Verification items for the finished model (mm, model axes). A direction names the side the tool comes from. Coordinates: 2 decimals unless noted, no trailing zeros. Write each loop counter-clockwise with the first axis right and the second up, starting at its lowest first coordinate (ties: lowest second). Pieces come first, ordered by that corner, then holes. Notation, with made-up numbers: (84, 88) -> (138, 88) arc R27 ccw to (138, 127) -> close; hole circle Ø3 at (18, 54.5). An arc over 180 degrees is marked (long way). Write item = value, one per line. Start each with the question number.
(1) Mould release check, pull along X, two halves, no side actions. Record for faces 4 (the face through (7, 35, 15)), 5 (the face through (0, 35, 15)), 6 (the face through (101, 36, 33.15)): released by +X, released by -X, zero draft, split by the parting line, or undercut.
(2) Material ranges on probe 1 along X at (y, z) = (58, 13); probe 2 along Z at (x, y) = (34.5, 14); probe 3 along Z at (x, y) = (4.5, 44), recorded low to high. Write a range as [from, to].
(3) Section check A-A (y = 28.5). Record the cut outline in (x, z).
(4) Section check B-B (z = 25). Record the cut outline in (x, y).
(5) Gauge pin test, flat end, axial feed: pin 1 Ø9 at (y, z) = (25.5, 13) entering from +X. Record the tip position at first contact, or that the pin passes through.
(6) Section check C-C (x = 142.5). Record the cut outline in (y, z).
(7) Section check D-D (z = 13). Record the cut outline in (x, y), plus the area to 3 significant figures.
(8) Set-up check for faces 1 (the face through (198, 35, 15)), 2 (the face through (205, 35, 15)), 3 (the face through (102, 0, 31)): record each of +Z, -Z, +X, -X, +Y, -Y from which the full face is reachable in a straight line by a thin tool's end or side.
```python
from build123d import *

# Parameters (mm, degrees)
SKETCH_1_W        = 7
SKETCH_1_H        = 70
EXTRUDE_1_DEPTH   = 30.15
EXTRUDE_1_2_DEPTH = 30.15
FILLET_1_R        = 30
FILLET_2_R        = 30
SKETCH_2_W        = 215.9
SKETCH_2_H        = 71
EXTRUDE_2_DEPTH   = 3
FILLET_3_R        = 3


with BuildPart() as part:
    # Sketch 1 → Extrude 1 (new body)
    with BuildSketch(Plane.XY):
        with Locations((3.5, 35)):
            Rectangle(SKETCH_1_W, SKETCH_1_H)
    extrude(amount=EXTRUDE_1_DEPTH)

    # Fillet 2
    fillet_2_edges = [part.edges().sort_by_distance(p)[0] for p in [
        (3.5, 70, 0),
    ]]
    fillet(fillet_2_edges, radius=FILLET_2_R)



with BuildPart() as body_2:
    # Sketch 1 → Extrude 1 2 (new body)
    with BuildSketch(Plane.XY):
        with Locations((201.5, 35)):
            Rectangle(SKETCH_1_W, SKETCH_1_H)
    extrude(amount=EXTRUDE_1_2_DEPTH)

    # Fillet 1
    fillet_1_edges = [body_2.edges().sort_by_distance(p)[0] for p in [
        (201.5, 70, 0),
    ]]
    fillet(fillet_1_edges, radius=FILLET_1_R)


with BuildPart() as part_1:
    add(part.part)

    add(body_2.part)  # Extrude 2 merges body 2
    # Sketch 2 → Extrude 2 (add)
    with BuildSketch(Plane.XY.offset(30.15)):
        with Locations((102.5, 35.5)):
            Rectangle(SKETCH_2_W, SKETCH_2_H)
    extrude(amount=EXTRUDE_2_DEPTH)

    # Fillet 3
    fillet_3_edges = [part_1.edges().sort_by_distance(p)[0] for p in [
        (210.45, 0, 31.65),
        (210.45, 71, 31.65),
        (-5.45, 71, 31.65),
        (-5.45, 0, 31.65),
    ]]
    fillet(fillet_3_edges, radius=FILLET_3_R)


solid = part_1.part
```
Response:
q1.face_4 = undercut
q1.face_5 = released by -X
q1.face_6 = zero draft
q2.probe_1 = [0, 7], [198, 205]
q2.probe_2 = [30.15, 33.15]
q2.probe_3 = [0.27, 33.15]
q3.outline = (-5.45, 30.15) -> (0, 30.15) -> (0, 0) -> (7, 0) -> (7, 30.15) -> (198, 30.15) -> (198, 0) -> (205, 0) -> (205, 30.15) -> (210.45, 30.15) -> (210.45, 33.15) -> (-5.45, 33.15) -> close
q4.outline = (0, 0) -> (7, 0) -> (7, 69.58) -> (0, 69.58) -> close; (198, 0) -> (205, 0) -> (205, 69.58) -> (198, 69.58) -> close
q5.pin_1 = 205
q6.outline = (0, 30.15) -> (71, 30.15) -> (71, 33.15) -> (0, 33.15) -> close
q7.outline = (0, 0) -> (7, 0) -> (7, 64.72) -> (0, 64.72) -> close; (198, 0) -> (205, 0) -> (205, 64.72) -> (198, 64.72) -> close
q7.area = 906 mm2
q8.face_1 = -Z, +Y, -Y
q8.face_2 = -Z, +X, +Y, -Y
q8.face_3 = +Z, -Z, +X, -X, -Y
